Design review of the part built by this model. Coordinates are the model's own, in mm. Face numbers are marked on the shaded views. Give positions to 0.01 mm unless a question says otherwise; leave off trailing zeros. Loops run counter-clockwise (first coordinate to the right, second up) from the corner with the lowest first, then second, coordinate; pieces in that order, holes last. Notation, with made-up numbers: M -6,-35 L 24,-35 A18 ccw 24,-23 Z; hole C 46.5,75 d2. An arc over 180 degrees is marked long. Use a Markdown table: item, result. Add a question column.
(1) Add section B-B, the plane x = 109. Give the boundary of the cut face in (y, z), then the cut area to 3 significant figures.
(2) Insertion check: pin 1 Ø12 at (x, y) = (120.5, 42.5) entering from -Z; pin 2 Ø4 at (y, z) = (1.5, -10) entering from +X; pin 3 Ø1 at (y, z) = (112.5, -6) entering from -X; pin 4 Ø3.5 at (x, y) = (25, 57) entering from -Z. Each pin has a flat end and moves straight along its axis. Give the tip position at first contact, or say it passes through.
(3) Add section C-C, the plane z = -8. Give the boundary of the cut face in (x, y), then the cut area to 3 significant figures.
(4) Add section A-A, the plane y = 57. Give the boundary of the cut face in (x, z), then the cut area to 3 significant figures.
(5) For probe 1 along Y at (x, z) = (114, -14.5); probe 2 along Y at (x, z) = (25, 4); probe 3 along Z at (x, y) = (86.5, 33.5), list the stretches that pass through material, from the lowest coordinate up.
(6) Add section D-D, the plane x = 44.5. Give the boundary of the cut face in (y, z).
(7) Draft analysis for pull direction Y (two halves, no side actions). For the marked faces 1, 2 and 3, state which applies: pulls with the +Y half, pulls with the -Y half, needs draft (parallel to the pull), parting line crosses it, or undercut.
```python
from build123d import *

# Parameters (mm, degrees)
SKETCH1_W           = 134
SKETCH1_H           = 114
BOSS_EXTRUDE1_DEPTH = 9.5
SKETCH2_W           = 115
SKETCH2_H           = 3.5
BOSS_EXTRUDE2_DEPTH = 20
SKETCH3_R           = 2.15
CUT_EXTRUDE1_DEPTH  = 179.387919995
SKETCH4_R           = 3.65
CUT_EXTRUDE2_DEPTH  = 3.6
CHAMFER1_SIZE       = 1
CHAMFER4_SIZE       = 0.5
SKETCH5_W           = 115
SKETCH5_H           = 1.75
BOSS_EXTRUDE3_DEPTH = 2
CHAMFER5_SIZE       = 0.5


with BuildPart() as part:
    # Sketch1 → Boss-Extrude1 (new body)
    with BuildSketch(Plane.XY):
        with Locations((67, 57)):
            Rectangle(SKETCH1_W, SKETCH1_H)
    extrude(amount=BOSS_EXTRUDE1_DEPTH)

    # Sketch2 → Boss-Extrude2 (add)
    with BuildSketch(Plane(origin=(0, 0, 0), x_dir=(-1, 0, 0), z_dir=(0, 0, -1))):
        Polygon((-67, 114), (-124.5, 114), (-124.5, 110.5), (-9.5, 110.5), (-9.5, 114), align=None)
        with Locations((-67, 1.75)):
            Rectangle(SKETCH2_W, SKETCH2_H)
    extrude(amount=BOSS_EXTRUDE2_DEPTH)

    # Sketch3 → Cut-Extrude1 (cut, through all)
    with BuildSketch(Plane.XY.offset(9.5)):
        with Locations((25, 57)):
            Circle(SKETCH3_R)
        with Locations((109, 57)):
            Circle(SKETCH3_R)
    extrude(amount=-CUT_EXTRUDE1_DEPTH, mode=Mode.SUBTRACT)

    # Sketch4 → Cut-Extrude2 (cut)
    with BuildSketch(Plane.XY.offset(9.5)):
        with Locations((25, 57)):
            Circle(SKETCH4_R)
        with Locations((109, 57)):
            Circle(SKETCH4_R)
    extrude(amount=-CUT_EXTRUDE2_DEPTH, mode=Mode.SUBTRACT)

    # Chamfer1
    chamfer1_edges = [part.edges().sort_by_distance(p)[0] for p in [
        (134, 57, 9.5),
        (67, 114, 9.5),
        (0, 57, 9.5),
        (67, 0, 9.5),
        (0, 114, 4.75),
        (134, 114, 4.75),
        (134, 0, 4.75),
        (0, 0, 4.75),
    ]]
    chamfer(chamfer1_edges, length=CHAMFER1_SIZE)

    # Chamfer4
    chamfer4_edges = [part.edges().sort_by_distance(p)[0] for p in [
        (21.35, 57, 9.5),
        (105.35, 57, 9.5),
    ]]
    chamfer(chamfer4_edges, length=CHAMFER4_SIZE)

    # Sketch5 → Boss-Extrude3 (add)
    with BuildSketch(Plane(origin=(0, 0, -20), x_dir=(-1, 0, 0), z_dir=(0, 0, -1))):
        with Locations((-67, 113.125)):
            Rectangle(SKETCH5_W, SKETCH5_H)
        with Locations((-67, 0.875)):
            Rectangle(SKETCH5_W, SKETCH5_H)
    extrude(amount=BOSS_EXTRUDE3_DEPTH)

    # Chamfer5
    chamfer5_edges = [part.edges().sort_by_distance(p)[0] for p in [
        (67, 114, -22),
        (67, 0, -22),
    ]]
    chamfer(chamfer5_edges, length=CHAMFER5_SIZE)


solid = part.part
```
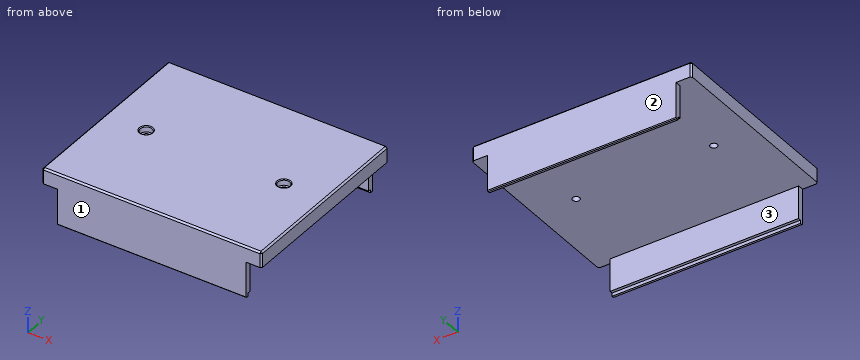
Established:
| question | item | result |
|---|---|---|
| 1 | outline | M 0,-21.5 L 0.5,-22 L 1.75,-22 L 1.75,-20 L 3.5,-20 L 3.5,0 L 54.85,0 L 54.85,5.9 L 53.35,5.9 L 53.35,9 L 52.85,9.5 L 1,9.5 L 0,8.5 Z; M 59.15,0 L 110.5,0 L 110.5,-20 L 112.25,-20 L 112.25,-22 L 113.5,-22 L 114,-21.5 L 114,8.5 L 113,9.5 L 61.15,9.5 L 60.65,9 L 60.65,5.9 L 59.15,5.9 Z |
| 1 | area | 1,180 mm^2 |
| 2 | pin 1 | z = 0 |
| 2 | pin 2 | x = 124.5 |
| 2 | pin 3 | x = 9.5 |
| 2 | pin 4 | through |
| 3 | outline | M 9.5,0 L 124.5,0 L 124.5,3.5 L 9.5,3.5 Z; M 9.5,110.5 L 124.5,110.5 L 124.5,114 L 9.5,114 Z |
| 3 | area | 805 mm^2 |
| 4 | outline | M 0,0 L 22.85,0 L 22.85,5.9 L 21.35,5.9 L 21.35,9 L 20.85,9.5 L 1,9.5 L 0,8.5 Z; M 27.15,0 L 106.85,0 L 106.85,5.9 L 105.35,5.9 L 105.35,9 L 104.85,9.5 L 29.15,9.5 L 28.65,9 L 28.65,5.9 L 27.15,5.9 Z; M 111.15,0 L 134,0 L 134,8.5 L 133,9.5 L 113.15,9.5 L 112.65,9 L 112.65,5.9 L 111.15,5.9 Z |
| 4 | area | 1,170 mm^2 |
| 5 | probe 1 | 0 to 3.5, 110.5 to 114 |
| 5 | probe 2 | 0 to 54.85, 59.15 to 114 |
| 5 | probe 3 | 0 to 9.5 |
| 6 | outline | M 0,-21.5 L 0.5,-22 L 1.75,-22 L 1.75,-20 L 3.5,-20 L 3.5,0 L 110.5,0 L 110.5,-20 L 112.25,-20 L 112.25,-22 L 113.5,-22 L 114,-21.5 L 114,8.5 L 113,9.5 L 1,9.5 L 0,8.5 Z |
| 7 | face 1 | pulls with the -Y half |
| 7 | face 2 | pulls with the +Y half |
| 7 | face 3 | undercut |
